from build123d import *

# Parameters (mm, degrees)
BOSS_EXTRUDE1_DEPTH = 10
BOSS_EXTRUDE2_DEPTH = 15


with BuildPart() as part:
    # Sketch1 → Boss-Extrude1 (new body)
    with BuildSketch(Plane.XY):
        with BuildLine():
            Line((-15, 25), (0, 25))
            Line((0, 25), (0, 0))
            Line((0, 0), (-30, 0))
            Line((-30, 0), (-30, 10))
            ThreePointArc((-30, 10), (-25.606601718, 20.606601718), (-15, 25))
        make_face()
    extrude(amount=BOSS_EXTRUDE1_DEPTH)

    # Sketch2 → Boss-Extrude2 (add)
    with BuildSketch(Plane.XY.offset(10)):
        with BuildLine():
            ThreePointArc((-30, 0), (-15, 15), (0, 0))
            ThreePointArc((0, 0), (-15, 6.771243445), (-30, 0))
        make_face()
    extrude(amount=BOSS_EXTRUDE2_DEPTH)


solid = part.part
Verification items for the finished model (mm, model axes). A direction names the side the tool comes from. Coordinates: 2 decimals unless noted, no trailing zeros. Write each loop counter-clockwise with the first axis right and the second up, starting at its lowest first coordinate (ties: lowest second). Pieces come first, ordered by that corner, then holes. Notation, with made-up numbers: (16.5, -15) -> (33.5, -15) arc R4 cw to (33.5, -11) -> close; hole circle Ø6 at (43.25, 10). An arc over 180 degrees is marked (long way). One line per item, written item: value. Start each with the question number.
Q1. Thickness scan on L1, parallel to Z at x = -13, y = 21.5; L2, parallel to Y at x = -14.5, z = 14.25 (3 decimals); L3, parallel to Y at x = -25, z = 7.75. Record the ranges inside material, lowest first. Write a range as from..to.
Q2. Cross-section at A-A on x = -6. Enter the section's corners in (y, z), and give its area (3 significant figures).
Q3. Cross-section at D-D on y = 17.5. Enter the section's corners in (x, z).
Q4. Go/stop test with flat-tipped pins: P1, Ø8, axis at x = -20.5, y = 21.5, coming from the +Z side; P2, Ø8, axis at x = -24, z = 12.5, coming from the +Y side; P3, Ø6, axis at y = 3, z = 21.5, coming from the -X side; P4, Ø3, axis at x = -5, z = 17.5, coming from the -Y side. Record where each tip stops, or that it passes through.
Q5. Mould release check, pull along X, two halves, no side actions. Record for faces 1 (the cylindrical face through (-15, 15, 17)), 2 (the flat face through (0, 13, 5)), 3 (the cylindrical face through (-25.72, 20.49, 4.93)), 4 (the cylindrical face through (-14.76, 6.77, 17.4)): pulls with the +X half, pulls with the -X half, needs draft (parallel to the pull), parting line crosses it, or undercut.
Q6. Cross-section at C-C on y = 11. Enter the section's corners in (x, z).
Q7. Access from +Z, -Z, +X, -X, +Y, -Y to the whole of each face (thin tool, end or side, straight path). Record for faces 5 (the flat face through (-15, 3, 10)), 6 (the flat face through (-8, 25, 5)).
Q8. Cross-section at B-B on z = 8.25. Enter the section's corners in (x, y), and give its area (3 significant figures).
Checked values:
1. L1: z = 0..10
1. L2: y = 6.765..14.992
1. L3: y = 0..21.18
2. outline: (0, 0) -> (25, 0) -> (25, 10) -> (12, 10) -> (12, 25) -> (4.63, 25) -> (4.63, 10) -> (0, 10) -> close
2. area: 361 mm²
3. outline: (-27.99, 0) -> (0, 0) -> (0, 10) -> (-27.99, 10) -> close
4. P1: stops at z = 10
4. P2: stops at y = 23.8
4. P3: stops at x = -30
4. P4: stops at y = 3.13
5. face 1: parting line crosses it
5. face 2: pulls with the +X half
5. face 3: pulls with the -X half
5. face 4: undercut
6. outline: (-29.97, 0) -> (0, 0) -> (0, 10) -> (-4.8, 10) -> (-4.8, 25) -> (-25.2, 25) -> (-25.2, 10) -> (-29.97, 10) -> close
7. face 5: +Z, -Y
7. face 6: +Z, -Z, +X, -X, +Y
8. outline: (-30, 0) -> (0, 0) -> (0, 25) -> (-15, 25) arc R15 ccw to (-30, 10) -> close
8. area: 702 mm²
